```python
from build123d import *

# Parameters (mm, degrees)
F0_R     = 15
F0_R_2   = 9.5
F0_R_3   = 7
F1_DEPTH = 7
F2_DEPTH = 20
F3_R     = 5
F4_SIZE  = 2
F5_SIZE  = 2


with BuildPart() as f1:
    # F0 (on Top) → F1 (new body)
    with BuildSketch(Plane.XY):
        Circle(F0_R)
        Circle(F0_R_2, mode=Mode.SUBTRACT)
        Circle(F0_R_2)
        Circle(F0_R_3, mode=Mode.SUBTRACT)
        Circle(F0_R_3)
    extrude(amount=F1_DEPTH)

    # F0 (on Top) → F2 (join)
    with BuildSketch(Plane.XY):
        Circle(F0_R_2)
        Circle(F0_R_3, mode=Mode.SUBTRACT)
    extrude(amount=F2_DEPTH)

    # F3
    f3_edges = [f1.edges().sort_by_distance(p)[0] for p in [
        (-9.5, 0, 7),
    ]]
    fillet(f3_edges, radius=F3_R)

    # F4
    f4_edges = [f1.edges().sort_by_distance(p)[0] for p in [
        (-7, 0, 20),
    ]]
    chamfer(f4_edges, length=F4_SIZE)

    # F5
    f5_edges = [f1.edges().sort_by_distance(p)[0] for p in [
        (-7, 0, 7),
    ]]
    chamfer(f5_edges, length=F5_SIZE)


solid = f1.part
```
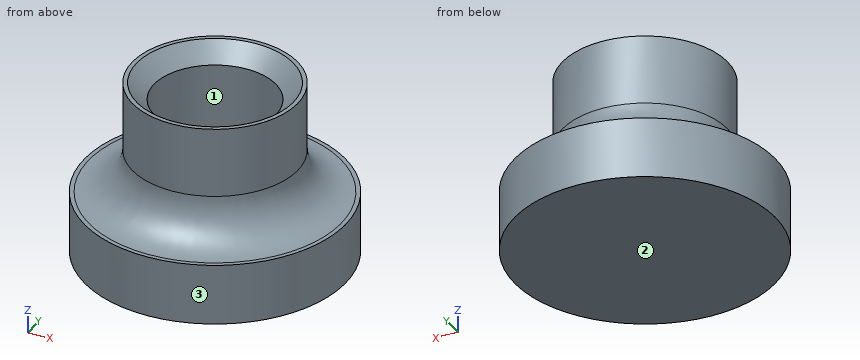
Work out the finished part from the listing and answer in its coordinate system (mm). Face numbers are marked on the shaded views. Give positions to 0.01 mm unless a question says otherwise; leave off trailing zeros. Order: outer loops, then holes, each group sorted by start corner. A loop starts at its lowest first (then second) coordinate and runs counter-clockwise, first axis right, second up. Notation, with made-up numbers: (59, -35) -> (65, -35) arc R21 ccw to (65, -26) -> close; hole circle Ø11 at (1, 85). An arc over 180 degrees is marked (long way). Answer as CSV lines item,"result". Start each with the question number.
(1) For a pull along Y with two mould halves and no side action, classify the marked faces 1, 2 and 3 as released by +Y, released by -Y, zero draft, split by the parting line, or undercut.
(2) Each of these flat-tipped pins is pushed along its axis until it touches: pin 1 Ø2 at (x, z) = (-6.5, 11) entering from +Y; pin 2 Ø5 at (x, z) = (-11, 7) entering from -Y; pin 3 Ø6 at (y, z) = (11, 15.5) entering from -X. Where does it stop, or does it pass through?
(3) Consider line 1 along Y through (x, z) = (0, 15.5); line 2 along X through (y, z) = (3.25, 14.5). Determine where each line is inside the solid, lowest interval first.
(4) Section D-D, the plane z = 6.5 is taken. Write down the section's boundary in (x, y), plus the area to 3 significant figures.
(5) Section C-C, the plane z = 12.5 is taken. Write down the section's boundary in (x, y).
(6) Section A-A, the plane x = 0 is taken. Write down the section's boundary in (y, z).
Entries:
1,face 1,"undercut"
1,face 2,"zero draft"
1,face 3,"split by the parting line"
2,pin 1,"y = 7.93"
2,pin 2,"y = -12.36"
2,pin 3,"x = -5.12"
3,line 1,"-9.5 to -7, 7 to 9.5"
3,line 2,"-8.93 to -6.2, 6.2 to 8.93"
4,outline,"circle Ø30 at (0, 0)"
4,area,"707 mm²"
5,outline,"circle Ø19 at (0, 0); hole circle Ø14 at (0, 0)"
6,outline,"(-15, 0) -> (15, 0) -> (15, 7) -> (14.5, 7) arc R5 cw to (9.5, 12) -> (9.5, 20) -> (9, 20) -> (7, 18) -> (7, 9) -> (5, 7) -> (-5, 7) -> (-7, 9) -> (-7, 18) -> (-9, 20) -> (-9.5, 20) -> (-9.5, 12) arc R5 cw to (-14.5, 7) -> (-15, 7) -> close"
